Autodesk Inventor part; units mm, degrees
ref_plane "YZ Plane" through (0, 0, 0) normal (1, 0, 0) x (0, 1, 0)
ref_plane "XZ Plane" through (0, 0, 0) normal (0, 1, 0) x (-1, 0, 0)
ref_plane "XY Plane" through (0, 0, 0) normal (0, 0, 1) x (1, 0, 0)
sketch "Sketch1" plane through (0, 0, 0) normal (0, 0, 1) x (1, 0, 0)
  arc A0 (3.1723, -7.3022) -> (10.7365, -7.3022) centre (6.9544, -6) ccw
  line L0 (1.6544, 0.1064) -> (1.6544, -2.5589)
  line L1 (1.6544, 0.1064) -> (12.2544, 0.1064)
  line L2 (12.2544, 0.1064) -> (12.2544, -2.5589)
  line L3 (1.7634, -3.21) -> (3.1723, -7.3022)
  line L4 (12.1455, -3.21) -> (10.7365, -7.3022)
  arc A1 (1.6544, -2.5589) -> (1.7634, -3.21) centre (3.6544, -2.5589) ccw
  arc A2 (12.1455, -3.21) -> (12.2544, -2.5589) centre (10.2544, -2.5589) ccw
  line L5 (12.0603, -7.7579) -> (13.4692, -3.6658)
  arc A3 (13.4692, -3.6658) -> (13.6544, -2.5589) centre (10.2544, -2.5589) ccw
  line L6 (13.6544, -2.5589) -> (13.6544, 1.5064)
  line L7 (13.6544, 1.5064) -> (1.2544, 1.5064)
  line L8 (0.2544, 0.5064) -> (0.2544, -2.5589)
  arc A4 (0.2544, -2.5589) -> (0.4396, -3.6658) centre (3.6544, -2.5589) ccw
  line L9 (0.4396, -3.6658) -> (1.8486, -7.7579)
  arc A5 (1.8486, -7.7579) -> (12.0603, -7.7579) centre (6.9544, -6) ccw
  arc A6 (1.2544, 1.5064) -> (0.2544, 0.5064) centre (1.2544, 0.5064) ccw
  point P0 (1.6544, -2.8936)
  point P1 (12.2544, -2.8936)
  point P2 (13.6544, 0.2)
  point P3 (12.7544, 1.5064)
  dimension "d12" = 4
  dimension "d13" = 3
  dimension "d14" = 3
  dimension "d16" = 2
  dimension "d17" = 1.4
  dimension "d18" = 1
  dimension "d35" = 10.6
extrude "Extrusion1" add sketch "Sketch1" along normal blind 2.5
sketch "Sketch3" plane through (1.6544, 0.1064, 2.5) normal (0, -1, 0) x (1, 0, 0)
  line L0 (10.2, 1) -> (12.4, 1)
  line L1 (12.9, 0.5) -> (12.9, -3)
  line L2 (12.4, -3.5) -> (10.2, -3.5)
  line L3 (9.7, -3) -> (9.7, 0.5)
  arc A0 (12.9, 0.5) -> (12.4, 1) centre (12.4, 0.5) ccw
  arc A1 (12.4, -3.5) -> (12.9, -3) centre (12.4, -3) ccw
  arc A2 (9.7, -3) -> (10.2, -3.5) centre (10.2, -3) ccw
  arc A3 (10.2, 1) -> (9.7, 0.5) centre (10.2, 0.5) ccw
  line L4 (-1.4, -2.5) -> (-1.4, 0)
  point P0 (9.7, 1)
  point P1 (12.9, -3.5)
  point P2 (12.9, 1)
  point P3 (9.7, -3.5)
  dimension "d21" = 4.5
  dimension "d22" = 3.2
  dimension "d27" = 0.5
  dimension "d36" = 11.1
extrude "Extrusion2" add sketch "Sketch3" against normal blind 3 draft -5
properties part number "fastener_01"
The model under review builds one solid part; all positions refer to its coordinate system, in mm. A direction names the side the tool comes from. Coordinates: 2 decimals unless noted, no trailing zeros. Write each loop counter-clockwise with the first axis right and the second up, starting at its lowest first coordinate (ties: lowest second). Pieces come first, ordered by that corner, then holes. Notation, with made-up numbers: (65.25, 84.25) - (115.25, 84.25) arc R30 cw to (115.25, 122.25) - close; hole circle Ø7 at (-31.75, -26.75). An arc over 180 degrees is marked (long way). Answer in a Markdown table with one row per item. Add a question column.
Q1. Clearance check with flat-ended pins moving along their axes: pin 1 (1.5 mm diameter, centred on x = 3, z = 0, fed in from +Y); pin 2 (4 mm diameter, centred on x = 7.5, y = -7, fed in from -Z); pin 3 (1.5 mm diameter, centred on y = 1.5, z = 1, fed in from -X); pin 4 (0.8 mm diameter, centred on y = -1.5, z = 1.5, fed in from +X). State where each tip first meets the part, or that it passes through.
Q2. To check wall thickness, follow line 1 along X through (y, z) = (-0.25, 0.1); line 2 along Y through (x, z) = (9, 0.6); line 3 along X through (y, z) = (-6, 0.25). State the ranges of each line that lie inside material, in increasing order. Write a range as from..to.
Q3. Consider section A-A on y = -0.5. Give the boundary of the cut face in (x, z), then the cut area to 3 significant figures.
Q4. Consider section B-B on z = 1.35. Give the boundary of the cut face in (x, y).
Q5. For faces 5 (the face through (2.46, -5.23, 1.23)), 6 (the face through (13.654, -1, 1)), 7 (the face through (6, 1.506, 1)), 8 (the face through (14.425, 1.585, 1.274)), 9 (the face through (1.134, -5.683, 1.232)), list the 3-axis set-ups (+Z, -Z, +X, -X, +Y, -Y) from which the entire face can be reached by the end or side of a thin tool; tool diameter is ignored.
Q6. Draft analysis for pull direction X (two halves, no side actions). For faces 1 (the face through (11.45, -5.23, 1.23)), 2 (the face through (1.654, -1, 1)), 3 (the face through (2, -5, 2.5)), 4 (the face through (7, -11.4, 1.2)), state which applies: +X half, -X half, draft (parallel to the pull), parting line (faces both ways), or undercut.
Q7. Consider section C-C on x = 8. Give the boundary of the cut face in (y, z).
Q8. Consider section D-D on y = 2. Give the boundary of the cut face in (x, z).
Answers below:
| question | item | result |
|---|---|---|
| 1 | pin 1 | y = 1.51 |
| 1 | pin 2 | through |
| 1 | pin 3 | x = 0.28 |
| 1 | pin 4 | x = 13.65 |
| 2 | line 1 | 0.25..1.65, 12.25..13.65 |
| 2 | line 2 | -11..-9.44, 0.11..1.51 |
| 2 | line 3 | 1.24..2.72, 11.18..12.67 |
| 3 | outline | (0.25, 0) - (1.65, 0) - (1.65, 2.5) - (0.25, 2.5) - close; (12.25, 0) - (13.65, 0) - (13.65, 2.5) - (12.25, 2.5) - close |
| 3 | area | 7.00 mm² |
| 4 | outline | (0.25, -2.56) arc R3.4 ccw to (0.44, -3.67) - (1.85, -7.76) arc R5.4 ccw to (12.06, -7.76) - (13.47, -3.67) arc R3.4 ccw to (13.65, -2.56) - (13.65, 0.11) - (14.55, 0.11) - (14.29, 3.11) - (11.62, 3.11) - (11.48, 1.51) - (1.25, 1.51) arc R1 ccw to (0.25, 0.51) - close; hole (1.65, -2.56) arc R2 ccw to (1.76, -3.21) - (3.17, -7.3) arc R4 ccw to (10.74, -7.3) - (12.15, -3.21) arc R2 ccw to (12.25, -2.56) - (12.25, 0.11) - (1.65, 0.11) - close |
| 5 | face 5 | +Z, -Z |
| 5 | face 6 | +Z, -Z, +X, -Y |
| 5 | face 7 | +Z, -Z, -X, +Y |
| 5 | face 8 | +Z, -Z, +X, +Y |
| 5 | face 9 | +Z, -Z, -X, -Y |
| 6 | face 1 | undercut |
| 6 | face 2 | undercut |
| 6 | face 3 | draft |
| 6 | face 4 | parting line |
| 7 | outline | (-11.3, 0) - (-9.86, 0) - (-9.86, 2.5) - (-11.3, 2.5) - close; (0.11, 0) - (1.51, 0) - (1.51, 2.5) - (0.11, 2.5) - close |
| 8 | outline | (11.52, -0.5) arc R0.33 ccw to (11.85, -0.83) - (14.05, -0.83) arc R0.33 ccw to (14.39, -0.5) - (14.39, 3) arc R0.33 ccw to (14.05, 3.33) - (11.85, 3.33) arc R0.33 ccw to (11.52, 3) - close |
